```python
from build123d import *

# Parameters (mm, degrees)
F1_DEPTH = 300
F2_R     = 13
F4_DEPTH = 18
F3_R     = 13
F5_DEPTH = 18


with BuildPart() as f1:
    # F0 (on Front) → F1 (new body)
    with BuildSketch(Plane.XZ):
        Polygon((-14.253071, 50.231077), (-49.253071, 50.231077), (-49.253071, -39.768923), (20.746929, -39.768923), (20.746929, -19.768923), (-14.253071, -19.768923), align=None)
    extrude(amount=F1_DEPTH)

    # F2 (on face) → F4 (cut)
    with BuildSketch(Plane.XY.offset(-19.768923)):
        with Locations((2.785809, -280.291462)):
            Circle(F2_R)
        with Locations((2.834997, -251.291504)):
            Circle(F2_R)
        with Locations((2.884185, -222.291546)):
            Circle(F2_R)
        with Locations((2.933373, -193.291588)):
            Circle(F2_R)
        with Locations((2.982561, -164.291629)):
            Circle(F2_R)
        with Locations((3.031749, -135.291671)):
            Circle(F2_R)
        with Locations((3.080937, -106.291713)):
            Circle(F2_R)
        with Locations((3.130125, -77.291754)):
            Circle(F2_R)
        with Locations((3.179313, -48.291796)):
            Circle(F2_R)
        with Locations((3.228501, -19.291838)):
            Circle(F2_R)
    extrude(amount=-F4_DEPTH, mode=Mode.SUBTRACT)

    # F3 (on face) → F5 (cut)
    with BuildSketch(Plane.XY.offset(50.231077)):
        with Locations((-32.380091, -282.027827)):
            Circle(F3_R)
        with Locations((-32.330904, -253.027869)):
            Circle(F3_R)
        with Locations((-32.281717, -224.027911)):
            Circle(F3_R)
        with Locations((-32.232531, -195.027952)):
            Circle(F3_R)
        with Locations((-32.183344, -166.027994)):
            Circle(F3_R)
        with Locations((-32.134158, -137.028036)):
            Circle(F3_R)
        with Locations((-32.084971, -108.028078)):
            Circle(F3_R)
        with Locations((-32.035784, -79.028119)):
            Circle(F3_R)
        with Locations((-31.986598, -50.028161)):
            Circle(F3_R)
        with Locations((-31.937411, -21.028203)):
            Circle(F3_R)
    extrude(amount=-F5_DEPTH, mode=Mode.SUBTRACT)


solid = f1.part
```
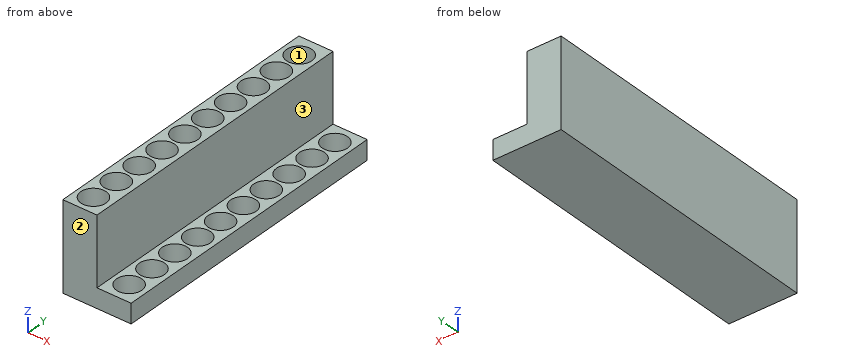
For this review, take the finished solid that the model builds, in its own axes (mm). Face numbers are marked on the shaded views. A direction names the side the tool comes from. Round coordinates to 2 decimals unless told otherwise and drop trailing zeros. Order: outer loops, then holes, each group sorted by start corner. A loop starts at its lowest first (then second) coordinate and runs counter-clockwise, first axis right, second up.
Q1. Wall thickness on line 1 (X direction, y = -220.5, z = -34); line 2 (Z direction, x = -45, y = -284); line 3 (Z direction, x = 1, y = -229.5): over which ranges is each line inside the solid? List them lowest first.
Findings below:
line 1: x = -49.25 to -9.99, 15.76 to 20.75
line 2: z = -39.77 to 32.23
line 3: z = -39.77 to -37.77
Q2. We need section A-A, the plane z = -26. State how many separate pieces and enclosed holes the cut face has, plus the area to 3 significant figures.
Findings below:
separate pieces: 1
enclosed holes: 10
area: 15,700 mm2
Q3. Insertion check: P1, Ø13, axis at x = 2, y = -161, coming from the +Z side; P2, Ø23.5, axis at x = -32.33, y = -253.03, coming from the +Z side; P3, Ø21, axis at x = 3.5, y = -44, coming from the +Z side. Each pin has a flat end and moves straight along its axis. Give the tip position at first contact, or say it passes through.
Findings below:
P1: stops at z = -37.77
P2: stops at z = 32.23
P3: stops at z = -19.77
Q4. We need section D-D, the plane y = -199.5. Give the boundary of the cut face in (x, z), plus the area to 3 significant figures.
Findings below:
outline: (-49.25, -39.77) - (20.75, -39.77) - (20.75, -19.77) - (14.36, -19.77) - (14.36, -37.77) - (-8.49, -37.77) - (-8.49, -19.77) - (-14.25, -19.77) - (-14.25, 50.23) - (-20.03, 50.23) - (-20.03, 32.23) - (-44.44, 32.23) - (-44.44, 50.23) - (-49.25, 50.23) - close
area: 3,000 mm2
Q5. Machinability: for the marked faces 1, 2 and 3, which of the approach directions +Z, -Z, +X, -X, +Y, -Y give a long, thin tool a straight path to every point of the face, cutting with its end or side? Answer none if there is none.
Findings below:
face 1: +Z
face 2: +Z, -Z, +X, -X, -Y
face 3: +Z, +X, +Y, -Y
Q6. We need section C-C, the plane z = -7.5. Give the boundary of the cut face in (x, y), plus the area to 3 significant figures.
Findings below:
outline: (-49.25, -300) - (-14.25, -300) - (-14.25, 0) - (-49.25, 0) - close
area: 10,500 mm2
Q7. We need section B-B, the plane y = -112.5. Give the boundary of the cut face in (x, z).
Findings below:
outline: (-49.25, -39.77) - (20.75, -39.77) - (20.75, -19.77) - (14.5, -19.77) - (14.5, -37.77) - (-8.34, -37.77) - (-8.34, -19.77) - (-14.25, -19.77) - (-14.25, 50.23) - (-19.88, 50.23) - (-19.88, 32.23) - (-44.29, 32.23) - (-44.29, 50.23) - (-49.25, 50.23) - close
